Check sheet for the modelled part. Datum: model origin and axes. Units: mm. A direction names the side the tool comes from. Coordinates: 2 decimals unless noted, no trailing zeros. Write each loop counter-clockwise with the first axis right and the second up, starting at its lowest first coordinate (ties: lowest second). Pieces come first, ordered by that corner, then holes. Notation, with made-up numbers: M 43.5,-37.75 L 82.5,-37.75 A27 ccw 82.5,-19.75 Z; hole C 44,13 d6. An arc over 180 degrees is marked long. Answer as CSV lines item,"result". Start each with the question number.
Q1. Access from +Z, -Z, +X, -X, +Y, -Y to the whole of each face (thin tool, end or side, straight path). Record for faces 1 (the flat face through (9, 64, 0)), 2 (the flat face through (33.918, 37.028, 0.021)).
Q2. Sectioned sample at D-D, the plane y = 29. Record the cut outline in (x, z), then the cut area to 3 significant figures.
Q3. Sectioned sample at B-B, the plane y = 70. Record the cut outline in (x, z), then the cut area to 3 significant figures.
Q4. Thickness scan on line 1 along Y through (x, z) = (-4, 0.65); line 2 along X through (y, z) = (74.8, 0.1) (3 decimals); line 3 along X through (y, z) = (52, 0.8). Record the ranges inside material, lowest first. Write a range as from..to.
Q5. Sectioned sample at C-C, the plane z = 0.55. Count the separate pieces of the cut face and the enclosed holes in it, then the cut area to 3 significant figures.
Q6. Mould release check, pull along X, two halves, no side actions. Record for faces 3 (the cylindrical face through (8.43, 28.6, -0.02)), 4 (the flat face through (-34.082, 36.572, 0.021)), 5 (the cylindrical face through (39.1, 0.86, 0.02)): pulls with the +X half, pulls with the -X half, needs draft (parallel to the pull), parting line crosses it, or undercut.
Q7. Depth check by flat-ended pin: pin 1 Ø1.5 at (y, z) = (36.5, -0.5) entering from -X (3 decimals); pin 2 Ø2.5 at (x, y) = (-27.5, 10) entering from +Z; pin 3 Ø1.5 at (y, z) = (38, 0) entering from -X. Enter the tip coordinate at first touch or a pass-through.
Q8. Sectioned sample at A-A, the plane x = -5.5. Record the cut outline in (y, z), then the cut area to 3 significant figures.
from build123d import *

# Parameters (mm, degrees)
EXTRUDE_1_DEPTH           = 1.5
SKETCH_2_W                = 18
SKETCH_2_H                = 18
CUT_EXTRUDE_1_DEPTH       = 3
FILLET_1_R                = 1
FILLET_2_R                = 2
FILLET_3_R                = 3
SKETCH_3_R                = 2.025
CUT_EXTRUDE_2_DEPTH       = 1
CUT_EXTRUDE_2_DEPTH_BACK  = 4
SKETCH_4_R                = 2.025
CUT_EXTRUDE_3_DEPTH       = 1
CUT_EXTRUDE_3_DEPTH_BACK  = 4
SKETCH_5_R                = 2.025
CUT_EXTRUDE_4_DEPTH       = 1
CUT_EXTRUDE_4_DEPTH_BACK  = 4
FILLET_4_R                = 3
EXTRUDE_2_DEPTH           = 3
FILLET_5_R                = 3
SKETCH_7_R                = 1.525
CUT_EXTRUDE_5_DEPTH       = 3
HOLE_WIZARD_1_D           = 4.05
HOLE_WIZARD_1_DEPTH       = 100
HOLE_WIZARD_1_CSINK_D     = 8
HOLE_WIZARD_1_CSINK_ANGLE = 90
EXTRUDE_3_DEPTH           = 3
FILLET_6_R                = 3
SKETCH_12_R               = 1.525
CUT_EXTRUDE_6_DEPTH       = 1
CUT_EXTRUDE_6_DEPTH_BACK  = 4
FILLET_7_R                = 2


with BuildPart() as part:
    # 草图1 → 凸台-拉伸1 (new body, symmetric)
    with BuildSketch(Plane.XY):
        Polygon((40, 0), (-40, 0), (-40, 20), (-15, 90), (15, 90), (40, 20), align=None)
    extrude(amount=EXTRUDE_1_DEPTH, both=True)

    # 草图2 → 切除-拉伸1 (cut)
    with BuildSketch(Plane.XY.offset(1.5)):
        Polygon((-15, 72.160717503), (-33.62882768, 20), (-15, 20), align=None)
        with Locations((0, 64)):
            Rectangle(SKETCH_2_W, SKETCH_2_H)
        with Locations((0, 37)):
            Rectangle(SKETCH_2_W, SKETCH_2_H)
    extrude(amount=-CUT_EXTRUDE_1_DEPTH, mode=Mode.SUBTRACT)

    # 圆角1
    fillet_1_edges = [part.edges().sort_by_distance(p)[0] for p in [
        (-15, 20, 0),
        (-15, 72.160717503, 0),
    ]]
    fillet(fillet_1_edges, radius=FILLET_1_R)

    # 圆角2
    fillet_2_edges = [part.edges().sort_by_distance(p)[0] for p in [
        (-9, 46, 0),
        (-9, 28, 0),
        (9, 28, 0),
        (9, 46, 0),
        (-9, 73, 0),
        (-9, 55, 0),
        (9, 55, 0),
        (9, 73, 0),
    ]]
    fillet(fillet_2_edges, radius=FILLET_2_R)

    # 圆角3
    fillet_3_edges = [part.edges().sort_by_distance(p)[0] for p in [
        (40, 0, 0),
        (-40, 0, 0),
        (-40, 20, 0),
        (-15, 90, 0),
        (15, 90, 0),
        (40, 20, 0),
    ]]
    fillet(fillet_3_edges, radius=FILLET_3_R)

    # 草图3 → 切除-拉伸2 (cut, two sides)
    with BuildSketch(Plane.XY.offset(1.5)) as cut_extrude_2_sk:
        with Locations((-27.5, 10)):
            Circle(SKETCH_3_R)
        with Locations((27.5, 10)):
            Circle(SKETCH_3_R)
    extrude(amount=CUT_EXTRUDE_2_DEPTH, mode=Mode.SUBTRACT)
    extrude(cut_extrude_2_sk.sketch, amount=-CUT_EXTRUDE_2_DEPTH_BACK, mode=Mode.SUBTRACT)

    # 草图4 → 切除-拉伸3 (cut, two sides)
    with BuildSketch(Plane.XY.offset(1.5)) as cut_extrude_3_sk:
        with Locations((0, 10)):
            Circle(SKETCH_4_R)
    extrude(amount=CUT_EXTRUDE_3_DEPTH, mode=Mode.SUBTRACT)
    extrude(cut_extrude_3_sk.sketch, amount=-CUT_EXTRUDE_3_DEPTH_BACK, mode=Mode.SUBTRACT)

    # 草图5 → 切除-拉伸4 (cut, two sides)
    with BuildSketch(Plane.XY.offset(1.5)) as cut_extrude_4_sk:
        with Locations((0, 24)):
            Circle(SKETCH_5_R)
        with Locations((0, 50.5)):
            Circle(SKETCH_5_R)
        with Locations((0, 81.5)):
            Circle(SKETCH_5_R)
    extrude(amount=CUT_EXTRUDE_4_DEPTH, mode=Mode.SUBTRACT)
    extrude(cut_extrude_4_sk.sketch, amount=-CUT_EXTRUDE_4_DEPTH_BACK, mode=Mode.SUBTRACT)

    # 圆角4
    fillet_4_edges = [part.edges().sort_by_distance(p)[0] for p in [
        (-33.62882768, 20, 0),
    ]]
    fillet(fillet_4_edges, radius=FILLET_4_R)

    # 草图6 → 凸台-拉伸2 (add)
    with BuildSketch(Plane(origin=(0, 0, -1.5), x_dir=(-1, 0, 0), z_dir=(0, 0, -1))):
        with BuildLine():
            Line((15, 66.387503754), (15, 50))
            Line((15, 50), (22.914541965, 50))
            Line((22.914541965, 50), (16.941741912, 66.723840151))
            ThreePointArc((16.941741912, 66.723840151), (15.82932767, 67.372831596), (15, 66.387503754))
        make_face()
        Polygon((-28, 78), (-28, 53.6), (-19.285714286, 78), align=None)
        Polygon((28, 78), (19.285714286, 78), (28, 53.6), align=None)
    extrude(amount=-EXTRUDE_2_DEPTH)

    # 圆角5
    fillet_5_edges = [part.edges().sort_by_distance(p)[0] for p in [
        (28, 53.6, 0),
        (-28, 78, 0),
        (19.285714286, 78, 0),
        (28, 78, 0),
        (-19.285714286, 78, 0),
        (-28, 53.6, 0),
    ]]
    fillet(fillet_5_edges, radius=FILLET_5_R)

    # 草图7 → 切除-拉伸5 (cut)
    with BuildSketch(Plane(origin=(0, 0, -1.5), x_dir=(-1, 0, 0), z_dir=(0, 0, -1))):
        with Locations((24.8, 74.8)):
            Circle(SKETCH_7_R)
        with Locations((24.8, 53.2)):
            Circle(SKETCH_7_R)
        with Locations((-24.8, 53.2)):
            Circle(SKETCH_7_R)
        with Locations((-24.8, 74.8)):
            Circle(SKETCH_7_R)
    extrude(amount=-CUT_EXTRUDE_5_DEPTH, mode=Mode.SUBTRACT)

    # 孔1
    with Locations(Plane.XY.offset(1.5)):
        with Locations((0, 81.5), (0, 50.5)):
            CounterSinkHole(HOLE_WIZARD_1_D / 2, HOLE_WIZARD_1_CSINK_D / 2, depth=HOLE_WIZARD_1_DEPTH, counter_sink_angle=HOLE_WIZARD_1_CSINK_ANGLE)

    # 草图11 → 凸台-拉伸3 (add)
    with BuildSketch(Plane.XY.offset(1.5)):
        with BuildLine():
            Line((12.885842411, 90), (28, 90))
            Line((28, 90), (28, 75))
            ThreePointArc((28, 75), (27.121320344, 77.121320344), (25, 78))
            Line((25, 78), (21.399871874, 78))
            ThreePointArc((21.399871874, 78), (19.671726564, 78.547753319), (18.57464614, 79.990990809))
            Line((18.57464614, 79.990990809), (15.711068146, 88.009009191))
            ThreePointArc((15.711068146, 88.009009191), (14.613987722, 89.452246681), (12.885842411, 90))
        make_face()
    extrude(amount=-EXTRUDE_3_DEPTH)

    # 圆角6
    fillet_6_edges = [part.edges().sort_by_distance(p)[0] for p in [
        (28, 90, 0),
    ]]
    fillet(fillet_6_edges, radius=FILLET_6_R)

    # 草图12 → 切除-拉伸6 (cut, two sides)
    with BuildSketch(Plane.XY.offset(1.5)) as cut_extrude_6_sk:
        with Locations((23.5, 86.5)):
            Circle(SKETCH_12_R)
        with Locations((23.5, 25.5)):
            Circle(SKETCH_12_R)
    extrude(amount=CUT_EXTRUDE_6_DEPTH, mode=Mode.SUBTRACT)
    extrude(cut_extrude_6_sk.sketch, amount=-CUT_EXTRUDE_6_DEPTH_BACK, mode=Mode.SUBTRACT)

    # 圆角7
    fillet_7_edges = [part.edges().sort_by_distance(p)[0] for p in [
        (-22.914541965, 50, 0),
        (-15, 50, 0),
    ]]
    fillet(fillet_7_edges, radius=FILLET_7_R)


solid = part.part
Output:
1,face 1,"+Z, -Z"
1,face 2,"+Z, -Z, +X, +Y"
2,outline,"M -36.79,-1.5 L -30.41,-1.5 L -30.41,1.5 L -36.79,1.5 Z; M -15,-1.5 L -8.73,-1.5 L -8.73,1.5 L -15,1.5 Z; M 8.73,-1.5 L 36.79,-1.5 L 36.79,1.5 L 8.73,1.5 Z"
2,area,"122 mm^2"
3,outline,"M -28,-1.5 L -9,-1.5 L -9,1.5 L -28,1.5 Z; M 9,-1.5 L 28,-1.5 L 28,1.5 L 9,1.5 Z"
3,area,"114 mm^2"
4,line 1,"y = 0..28, 46..55, 73..90"
4,line 2,"x = -28..-26.325, -23.275..23.275, 26.325..28"
4,line 3,"x = -28.57..-25.74, -23.86..-2.94, 2.94..23.86, 25.74..28.57"
5,separate pieces,"1"
5,enclosed holes,"15"
5,area,"4,600 mm^2"
6,face 3,"undercut"
6,face 4,"pulls with the -X half"
6,face 5,"pulls with the +X half"
7,pin 1,"stops at x = -34.375"
7,pin 2,"passes through"
7,pin 3,"stops at x = -33.84"
8,outline,"M 0,-1.5 L 28,-1.5 L 28,1.5 L 0,1.5 Z; M 46,-1.5 L 55,-1.5 L 55,1.5 L 46,1.5 Z; M 73,-1.5 L 90,-1.5 L 90,1.5 L 73,1.5 Z"
8,area,"162 mm^2"
